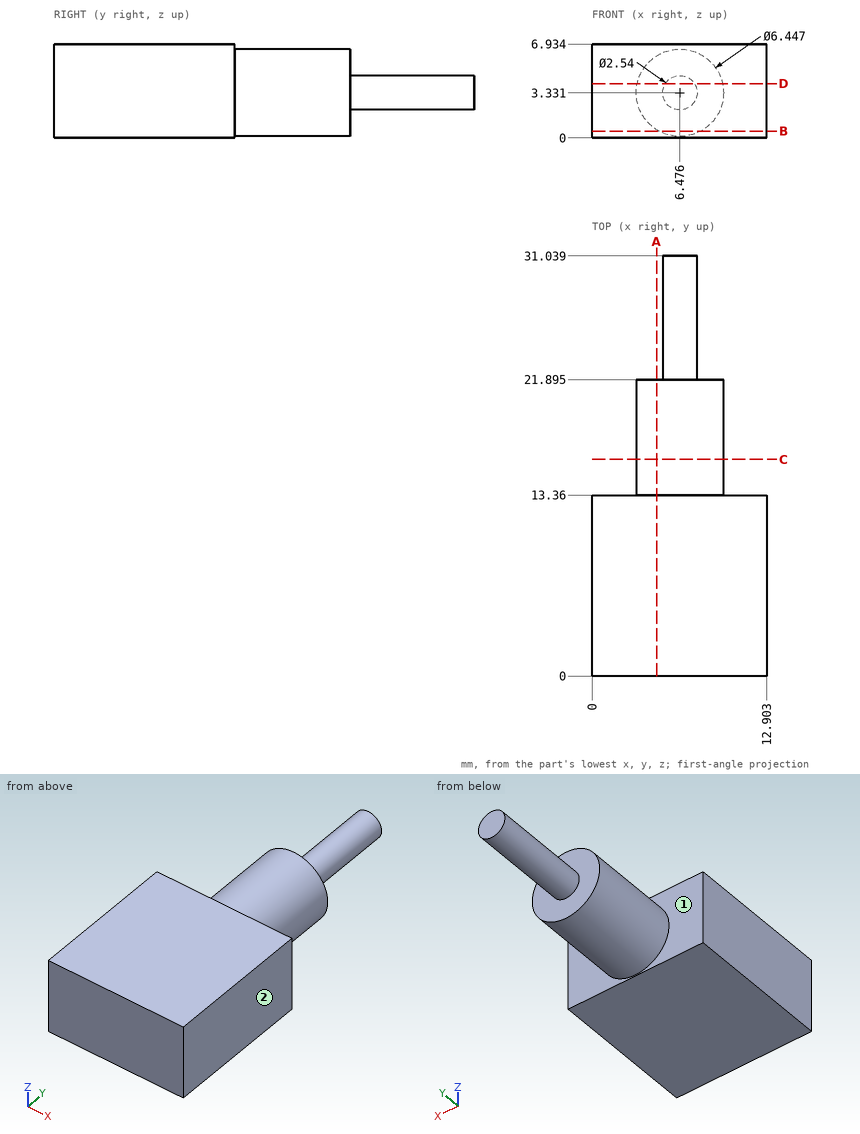
Part print with two shaded views. Sizes in mm from the minimum x, y, z corner. A direction names the side the tool comes from. Give positions to 0.01 mm unless a question says otherwise; leave off trailing zeros. Order: outer loops, then holes, each group sorted by start corner. A loop starts at its lowest first (then second) coordinate and runs counter-clockwise, first axis right, second up. Notation, with made-up numbers: (63, 5.5) - (84, 5.5) arc R10 ccw to (84, 10.5) - close; hole circle Ø5 at (39.5, -26). An arc over 180 degrees is marked (long way). Write each question's results on one line, items separated by ' | '.
1. Saw through at A-A on x = 4.75. List the corners of the cut face in (y, z) (1 decimal).
Calculated:
outline: (0, 0) - (13.4, 0) - (13.4, 0.6) - (21.9, 0.6) - (21.9, 6.1) - (13.4, 6.1) - (13.4, 6.9) - (0, 6.9) - close
2. Saw through at C-C on y = 16. List the corners of the cut face in (x, z).
Calculated:
outline: circle Ø6.45 at (6.48, 3.33)
3. Saw through at B-B on z = 0.5. List the corners of the cut face in (x, y) (1 decimal), and give its area (3 significant figures).
Calculated:
outline: (0, 0) - (12.9, 0) - (12.9, 13.4) - (8, 13.4) - (8, 21.9) - (4.9, 21.9) - (4.9, 13.4) - (0, 13.4) - close | area: 199 mm2
4. Probe L1, parallel to Y at x = 7.25, z = 1 (1 decimal); L2, parallel to Y at x = 1.75, z = 0.5; L3, parallel to X at y = 26.5, z = 3. List the from-to ranges inside material, lowest first. Write a range as from..to.
Calculated:
L1: y = 0..21.9 | L2: y = 0..13.36 | L3: x = 5.25..7.7
5. 3-axis set-ups, long thin cutter, end or side, ignore diameter. For the marked faces 1 and 2: which of +Z, -Z, +X, -X, +Y, -Y reach the whole face in a straight line?
Calculated:
face 1: +Y | face 2: +Z, -Z, +X, +Y, -Y
6. Pin check, flat tips, straight feed: pin 1 (1.5 mm diameter, centred on y = 19, z = 2, fed in from -X) (1 decimal); pin 2 (4 mm diameter, centred on y = 26.5, z = 4, fed in from -X). Stop position of each tip, or through.
Calculated:
pin 1: stops at x = 3.3 | pin 2: stops at x = 5.21
7. Saw through at D-D on z = 4. List the corners of the cut face in (x, y) (1 decimal), and give its area (3 significant figures).
Calculated:
outline: (0, 0) - (12.9, 0) - (12.9, 13.4) - (9.6, 13.4) - (9.6, 21.9) - (7.6, 21.9) - (7.6, 31) - (5.4, 31) - (5.4, 21.9) - (3.3, 21.9) - (3.3, 13.4) - (0, 13.4) - close | area: 246 mm2
